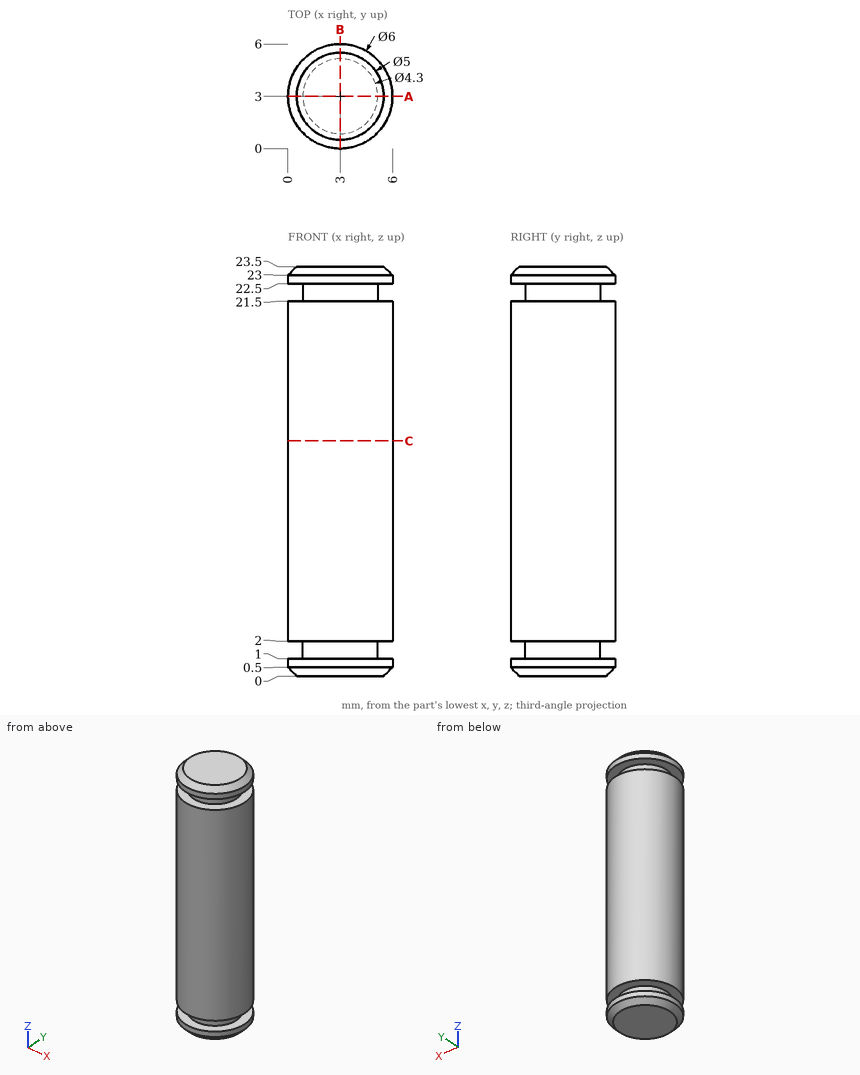
Drawing for the job (mm, zero at the part's lowest x, y, z). Round coordinates to 2 decimals unless told otherwise and drop trailing zeros. Loops run counter-clockwise (first coordinate to the right, second up) from the corner with the lowest first, then second, coordinate; pieces in that order, holes last. Notation, with made-up numbers: (48, 73.5) -> (91, 73.5) arc R15 ccw to (91, 83.5) -> close; hole circle Ø1 at (55.25, 26.25). An arc over 180 degrees is marked (long way). Answer as CSV lines item,"result". Start each with the question number.
1) Slice it at A-A (y = 3). List the corners of the cut face in (x, z).
2) Probe line 1 along Z through (x, y) = (1.1, 1.5); line 2 along Z through (x, y) = (5.2, 4.9); line 3 along X through (y, z) = (1.6, 8.5). List the from-to ranges inside material, lowest first.
3) Pin check, flat tips, straight feed: P1, Ø3, axis at y = 1, z = 18, coming from the -X side; P2, Ø1, axis at y = 1, z = 20.5, coming from the +X side; P3, Ø1.5, axis at x = 2, z = 7.5, coming from the -Y side. Stop position of each tip, or through.
4) Slice it at C-C (z = 13.5). List the corners of the cut face in (x, y), plus the area to 3 significant figures.
Filled in:
1,outline,"(0, 0.5) -> (0.5, 0) -> (5.5, 0) -> (6, 0.5) -> (6, 1) -> (5.15, 1) -> (5.15, 2) -> (6, 2) -> (6, 21.5) -> (5.15, 21.5) -> (5.15, 22.5) -> (6, 22.5) -> (6, 23) -> (5.5, 23.5) -> (0.5, 23.5) -> (0, 23) -> (0, 22.5) -> (0.85, 22.5) -> (0.85, 21.5) -> (0, 21.5) -> (0, 2) -> (0.85, 2) -> (0.85, 1) -> (0, 1) -> close"
2,line 1,"z = 0 to 1, 2 to 21.5, 22.5 to 23.5"
2,line 2,"z = 0.41 to 1, 2 to 21.5, 22.5 to 23.09"
2,line 3,"x = 0.35 to 5.65"
3,P1,"stops at x = 0.04"
3,P2,"stops at x = 5.6"
3,P3,"stops at y = 0.01"
4,outline,"circle Ø6 at (3, 3)"
4,area,"28.3 mm2"
